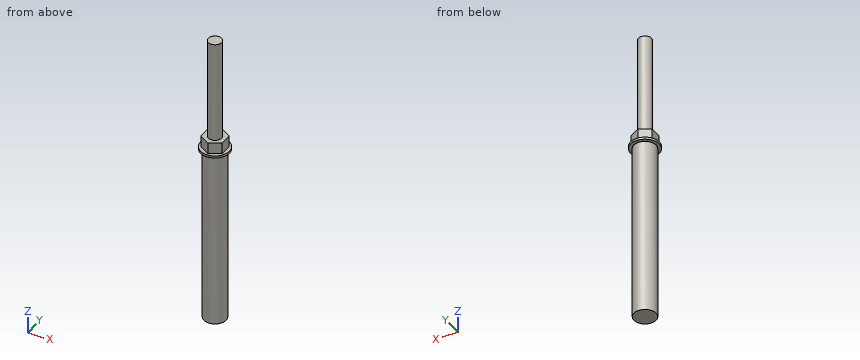
from build123d import *

# Parameters (mm, degrees)
SKETCH1_R           = 5
BOSS_EXTRUDE1_DEPTH = 80
SKETCH2_R           = 6.5
BOSS_EXTRUDE2_DEPTH = 1
BOSS_EXTRUDE5_DEPTH = 5
SKETCH6_R           = 3.019653564
BOSS_EXTRUDE6_DEPTH = 45.5


with BuildPart() as part:
    # Sketch1 → Boss-Extrude1 (new body)
    with BuildSketch(Plane.XY):
        Circle(SKETCH1_R)
    extrude(amount=BOSS_EXTRUDE1_DEPTH)

    # Sketch2 → Boss-Extrude2 (add)
    with BuildSketch(Plane.XY.offset(80)):
        Circle(SKETCH2_R)
    extrude(amount=BOSS_EXTRUDE2_DEPTH)

    # Sketch5 → Boss-Extrude5 (add)
    with BuildSketch(Plane.XY.offset(81)):
        Polygon((4.778851136, -2.820156932), (4.831753114, 2.728528019), (0.052901978, 5.548684951), (-4.778851136, 2.820156932), (-4.831753114, -2.728528019), (-0.052901978, -5.548684951), align=None)
    extrude(amount=BOSS_EXTRUDE5_DEPTH)

    # Sketch6 → Boss-Extrude6 (add)
    with BuildSketch(Plane.XY.offset(86)):
        Circle(SKETCH6_R)
    extrude(amount=BOSS_EXTRUDE6_DEPTH)


solid = part.part
Read the model definition and answer for the solid it produces. Units are mm, in the model's axes. Coordinates: 2 decimals unless noted, no trailing zeros. Loops run counter-clockwise (first coordinate to the right, second up) from the corner with the lowest first, then second, coordinate; pieces in that order, holes last. Notation, with made-up numbers: (-36.75, -27) -> (-29.75, -27) arc R11 cw to (-29.75, -9) -> close; hole circle Ø10 at (13.5, 27). An arc over 180 degrees is marked (long way). Write item = value, one per line. Start each with the question number.
1) Given P1, Ø4, axis at x = 2.5, y = -5, coming from the +Z side; P2, Ø3, axis at y = -4.5, z = 62, coming from the +X side; P3, Ø4, axis at x = 4, z = 63.5, coming from the +Y side; P4, Ø6, axis at x = -1.5, y = -1, coming from the -Z side, each flat-ended and moving along its own axis, determine where each tip first touches the part or whether it passes through.
2) Find the intervals of material crossed by L1, parallel to Z at x = 5.5, y = -2.75; L2, parallel to X at y = -4, z = 14; L3, parallel to Z at x = -1.75, y = -2.5, in increasing order. Write a range as from..to.
3) The part is cut by section B-B, the plane z = 118. Determine the outline of the cut face in (x, y), plus the area to 3 significant figures.
4) The part is cut by section A-A, the plane y = 0. Determine the outline of the cut face in (x, z).
5) The part is cut by section C-C, the plane z = 26. Determine the outline of the cut face in (x, y).
Result:
q1.P1 = 86
q1.P2 = 4
q1.P3 = 4.58
q1.P4 = 0
q2.L1 = 80..81
q2.L2 = -3..3
q2.L3 = 0..86
q3.outline = circle Ø6.04 at (0, 0)
q3.area = 28.6 mm²
q4.outline = (-6.5, 80) -> (-5, 80) -> (-5, 0) -> (5, 0) -> (5, 80) -> (6.5, 80) -> (6.5, 81) -> (4.81, 81) -> (4.81, 86) -> (3.02, 86) -> (3.02, 131.5) -> (-3.02, 131.5) -> (-3.02, 86) -> (-4.81, 86) -> (-4.81, 81) -> (-6.5, 81) -> close
q5.outline = circle Ø10 at (0, 0)
